CAD build for the part. Positions are in the model's coordinates, mm. A direction names the side the tool comes from. Give positions to 0.01 mm unless a question says otherwise; leave off trailing zeros. Loops run counter-clockwise (first coordinate to the right, second up) from the corner with the lowest first, then second, coordinate; pieces in that order, holes last. Notation, with made-up numbers: M -23,50.5 L 14,50.5 A18 ccw 14,62.5 Z; hole C -7.75,-2 d1. An arc over 180 degrees is marked long. One line per question, with ' | ' between items.
```python
from build123d import *

# Parameters (mm, degrees)
F2_R     = 3.5
F2_R_2   = 1.5
F3_DEPTH = 7
F4_SIZE  = 1
F5_R     = 2
F6_R     = 0.5


with BuildPart() as f1:
    # F0 (on Right) → F1 (revolve)
    with BuildSketch(Plane.YZ):
        Polygon((-8.5, 7), (-8.5, 0), (-6.5, 0), (-6.5, 5), (-6, 5), (-6, 5.5), (0, 5.5), (0, 7), align=None)
    revolve(axis=Axis((0, 0, 6.25), (0, 0, -1)))

    # F2 (on Top) → F3 (join)
    with BuildSketch(Plane.XY):
        with Locations((0, 11)):
            Circle(F2_R)
        with Locations((0, 11)):
            Circle(F2_R_2, mode=Mode.SUBTRACT)
        with Locations((-9.5262794416, -5.5)):
            Circle(F2_R)
        with Locations((-9.5262794416, -5.5)):
            Circle(F2_R_2, mode=Mode.SUBTRACT)
        with Locations((9.5262794416, -5.5)):
            Circle(F2_R)
        with Locations((9.5262794416, -5.5)):
            Circle(F2_R_2, mode=Mode.SUBTRACT)
    extrude(amount=F3_DEPTH)

    # F4
    f4_edges = [f1.edges().sort_by_distance(p)[0] for p in [
        (-1.5, 11, 7),
        (-11.026279, -5.5, 7),
        (8.026279, -5.5, 7),
    ]]
    chamfer(f4_edges, length=F4_SIZE)

    # F5
    f5_edges = [f1.edges().sort_by_distance(p)[0] for p in [
        (-2.13588, 8.227273, 3.5),
        (2.13588, 8.227273, 3.5),
        (-6.057087, -5.963363, 3.5),
        (-8.192967, -2.26391, 3.5),
        (6.057087, -5.963363, 3.5),
        (8.192967, -2.26391, 3.5),
    ]]
    fillet(f5_edges, radius=F5_R)

    # F6
    f6_edges = [f1.edges().sort_by_distance(p)[0] for p in [
        (0, -8.5, 7),
        (-5.660825, -7.077944, 7),
        (-8.960092, -1.363447, 7),
        (-12.557368, -7.25, 7),
        (-7.361216, 4.25, 7),
        (-3.299266, 8.44139, 7),
        (3.299266, 8.44139, 7),
        (0, 14.5, 7),
        (7.361216, 4.25, 7),
        (5.660825, -7.077944, 7),
        (8.960092, -1.363447, 7),
        (12.557368, -7.25, 7),
    ]]
    fillet(f6_edges, radius=F6_R)


solid = f1.part
```
Item 1: Drill centre lines: line 1 along X through (y, z) = (0, 5.45); line 2 along Y through (x, z) = (-1.25, 4.25); line 3 along X through (y, z) = (-4.75, 4). Where is each one in solid material? Low to high. Write a range as [from, to].
Conclusion:
line 1: [-8.5, -6], [6, 8.5] | line 2: [-8.41, -6.38], [6.38, 10.17], [11.83, 14.27] | line 3: [-12.94, -10.83], [-8.23, -4.44], [4.44, 8.23], [10.83, 12.94]
Item 2: 3-axis set-ups, long thin cutter, end or side, ignore diameter. For faces 1 (the cylindrical face through (3.955, 5.158, 2.535)), 2 (the cylindrical face through (12.51, -7.33, 3.2)): which of +Z, -Z, +X, -X, +Y, -Y reach the whole face in a straight line?
Conclusion:
face 1: -Z | face 2: +Z, -Z
Item 3: Saw through at D-D on z = 4.5. State how many separate pieces and enclosed holes the cut face has, and give its area (3 significant figures).
Conclusion:
separate pieces: 1 | enclosed holes: 4 | area: 186 mm²
Item 4: Saw through at A-A on x = 0. Give the cut face in (y, z), and give its area (3 significant figures).
Conclusion:
outline: M -8.5,0 L -6.5,0 L -6.5,5 L -6,5 L -6,5.5 L 6,5.5 L 6,5 L 6.5,5 L 6.5,0 L 9.5,0 L 9.5,6 L 8.5,7 L -8,7 A0.5 ccw -8.5,6.5 Z; M 12.5,0 L 14.5,0 L 14.5,6.5 A0.5 ccw 14,7 L 13.5,7 L 12.5,6 Z | area: 67.9 mm²
Item 5: Saw through at C-C on y = -5.5. Give the cut face in (x, z), and give its area (3 significant figures).
Conclusion:
outline: M -13.03,0 L -11.03,0 L -11.03,6 L -12.03,7 L -12.53,7 A0.5 ccw -13.03,6.5 Z; M -8.03,0 L -3.46,0 L -3.46,5 L -2.4,5 L -2.4,5.5 L 2.4,5.5 L 2.4,5 L 3.46,5 L 3.46,0 L 8.03,0 L 8.03,6 L 7.03,7 L -7.03,7 L -8.03,6 Z; M 11.03,0 L 13.03,0 L 13.03,6.5 A0.5 ccw 12.53,7 L 12.03,7 L 11.03,6 Z | area: 101 mm²
Item 6: Mould opens along X. For faces 3 (the flat face through (0, 0, 7)), 4 (the cylindrical face through (7.33, 4.3, 3.2)), 5 (the flat face through (6, -2, 5)) say: pulls with the +X half, pulls with the -X half, needs draft (parallel to the pull), parting line crosses it, or undercut.
Conclusion:
face 3: needs draft | face 4: pulls with the +X half | face 5: undercut
Item 7: Saw through at B-B on y = 11. Give the cut face in (x, z).
Conclusion:
outline: M -3.5,0 L -1.5,0 L -1.5,6 L -2.5,7 L -3,7 A0.5 ccw -3.5,6.5 Z; M 1.5,0 L 3.5,0 L 3.5,6.5 A0.5 ccw 3,7 L 2.5,7 L 1.5,6 Z
Item 8: Drop flat-ended pins along their axis: P1, Ø5, axis at x = -9.53, y = -5.5, coming from the -Z side; P2, Ø11, axis at x = 0, y = 0, coming from the -Z side; P3, Ø3, axis at x = 8, z = 3.5, coming from the +Y side; P4, Ø4, axis at x = -7, z = 1.5, coming from the -Y side. Give the stop position or say it passes through.
Conclusion:
P1: z = 0 | P2: z = 5.5 | P3: y = 5.48 | P4: y = -8.96
